```python
from build123d import *

# Parameters (mm, degrees)
SKETCH2_W           = 15
SKETCH2_H           = 7.5
SKETCH3_R           = 2.7
CUT_EXTRUDE1_DEPTH  = 10
SKETCH5_R           = 1.6
CUT_EXTRUDE2_DEPTH  = 11
SKETCH6_W           = 7
SKETCH6_H           = 7
BOSS_EXTRUDE1_DEPTH = 5
SKETCH7_W           = 4.9
SKETCH7_H           = 4.9
BOSS_EXTRUDE2_DEPTH = 15.3
SKETCH8_W           = 7
SKETCH8_H           = 7
BOSS_EXTRUDE3_DEPTH = 1


with BuildPart() as part:
    # Sketch2 → Revolve1 (revolve)
    with BuildSketch(Plane.XY):
        with Locations((7.5, 3.75)):
            Rectangle(SKETCH2_W, SKETCH2_H)
    revolve(axis=Axis((15, 0, 0), (-1, 0, 0)))

    # Sketch3 → Cut-Extrude1 (cut)
    with BuildSketch(Plane(origin=(15, 0, 0), x_dir=(0, 0, -1), z_dir=(1, 0, 0))):
        Circle(SKETCH3_R)
    extrude(amount=-CUT_EXTRUDE1_DEPTH, mode=Mode.SUBTRACT)

    # Sketch5 → Cut-Extrude2 (cut)
    with BuildSketch(Plane(origin=(0, 0, 0), x_dir=(1, 0, 0), z_dir=(0, 1, 0))):
        with Locations((7, 0)):
            Circle(SKETCH5_R)
    extrude(amount=CUT_EXTRUDE2_DEPTH, mode=Mode.SUBTRACT)

    # Sketch6 → Boss-Extrude1 (add)
    with BuildSketch(Plane.ZY):
        Rectangle(SKETCH6_W, SKETCH6_H)
    extrude(amount=BOSS_EXTRUDE1_DEPTH)

    # Sketch7 → Boss-Extrude2 (add)
    with BuildSketch(Plane.ZY.offset(5)):
        Rectangle(SKETCH7_W, SKETCH7_H)
    extrude(amount=BOSS_EXTRUDE2_DEPTH)

    # Sketch8 → Boss-Extrude3 (add)
    with BuildSketch(Plane.ZY.offset(20.3)):
        Rectangle(SKETCH8_W, SKETCH8_H)
    extrude(amount=BOSS_EXTRUDE3_DEPTH)


solid = part.part
```
Here's how the part is built. I have some questions about the finished solid (model axes, mm). A direction names the side the tool comes from. Coordinates: 2 decimals unless noted, no trailing zeros. Loops run counter-clockwise (first coordinate to the right, second up) from the corner with the lowest first, then second, coordinate; pieces in that order, holes last. Notation, with made-up numbers: (79, -18.75) - (118, -18.75) arc R33 ccw to (118, 15.25) - close; hole circle Ø9 at (58, 67). An arc over 180 degrees is marked (long way). Return JSON: item names as keys, results as strings. Group by question number.
Item 1: If we section it at B-B on y = 0: Write out the boundary of the cut face in (x, z), and give its area (3 significant figures).
Item 2: Will these pins go through, and if not, where does the flat tip stop? P1, Ø1, axis at x = -15, z = -3.5, coming from the +Y side; P2, Ø2.5, axis at x = -9.5, y = 0, coming from the -Z side; P3, Ø5, axis at x = -17.5, y = -1.5, coming from the +Z side; P4, Ø1, axis at x = -3.5, z = 3.5, coming from the +Y side.
Item 3: On a 3-axis mill with a long thin cutter (end or side, diameter ignored), from which of +Z, -Z, +X, -X, +Y, -Y can I reach the whole of each face in a straight line? I mean faces 4 (the face through (-21, 0, 3.5)), 5 (the face through (-5, 0, -3)), 6 (the face through (-13, 0, 2.45)), 7 (the face through (-2, 3.5, 0)), 8 (the face through (5, 0, 0)). Say none if no direction works.
Item 4: I need wall thicknesses on line 1 (Y direction, x = 9, z = 0); line 2 (X direction, y = 4.8, z = 0); line 3 (Y direction, x = 8, z = 0). Which ranges of each line are inside material? Lowest first, please. Write a range as from..to.
Item 5: If we section it at A-A on z = 0: Write out the boundary of the cut face in (x, y).
Item 6: We'd pull the mould along X, two halves only. Please class faces 1 (the face through (15, 0, 3)), 2 (the face through (-2, 0, 3.5)), 3 (the face through (-13, -2.45, 0)): +X half, -X half, draft (parallel to the pull), parting line (faces both ways), or undercut.
Item 7: If we section it at D-D on x = 10: Write out the boundary of the cut face in (y, z), and give its area (3 significant figures).
Item 8: If we section it at C-C on x = -10.5: Write out the boundary of the cut face in (y, z).
Calculated:
{
 "1": {"outline": "(-21.3, -3.5) - (-20.3, -3.5) - (-20.3, -2.45) - (-5, -2.45) - (-5, -3.5) - (0, -3.5) - (0, -7.5) - (15, -7.5) - (15, -2.7) - (5, -2.7) - (5, 2.7) - (15, 2.7) - (15, 7.5) - (0, 7.5) - (0, 3.5) - (-5, 3.5) - (-5, 2.45) - (-20.3, 2.45) - (-20.3, 3.5) - (-21.3, 3.5) - close", "area": "288 mm^2"},
 "2": {"P1": "passes through", "P2": "stops at z = -2.45", "P3": "stops at z = 2.45", "P4": "stops at y = 3.5"},
 "3": {"face 4": "+Z, -X, +Y, -Y", "face 5": "none", "face 6": "+Z, +Y, -Y", "face 7": "+Z, -Z, -X, +Y", "face 8": "+X"},
 "4": {"line 1": "y = -7.5..-2.7, 2.7..7.5", "line 2": "x = 0..5.4, 8.6..15", "line 3": "y = -7.5..-2.7"},
 "5": {"outline": "(-21.3, -3.5) - (-20.3, -3.5) - (-20.3, -2.45) - (-5, -2.45) - (-5, -3.5) - (0, -3.5) - (0, -7.5) - (15, -7.5) - (15, -2.7) - (5, -2.7) - (5, 2.7) - (5.4, 2.7) - (5.4, 7.5) - (0, 7.5) - (0, 3.5) - (-5, 3.5) - (-5, 2.45) - (-20.3, 2.45) - (-20.3, 3.5) - (-21.3, 3.5) - close; (8.6, 2.7) - (15, 2.7) - (15, 7.5) - (8.6, 7.5) - close"},
 "6": {"face 1": "+X half", "face 2": "draft", "face 3": "undercut"},
 "7": {"outline": "circle Ø15 at (0, 0); hole circle Ø5.4 at (0, 0)", "area": "154 mm^2"},
 "8": {"outline": "(-2.45, -2.45) - (2.45, -2.45) - (2.45, 2.45) - (-2.45, 2.45) - close"}
}
